from build123d import *

# Parameters (mm, degrees)
SKETCH1_W           = 80
SKETCH1_H           = 15
BOSS_EXTRUDE1_DEPTH = 5
FILLET1_R           = 6
SKETCH3_W           = 20
SKETCH3_H           = 15
CUT_EXTRUDE2_DEPTH  = 2.5
CUT_EXTRUDE3_DEPTH  = 2
SKETCH5_R           = 1.25
CUT_EXTRUDE4_DEPTH  = 41.807474805
SKETCH6_R           = 2.5
CUT_EXTRUDE5_DEPTH  = 1.5
SKETCH7_R           = 3.677678073
CUT_EXTRUDE6_DEPTH  = 1


with BuildPart() as part:
    # Sketch1 → Boss-Extrude1 (new body)
    with BuildSketch(Plane(origin=(0, 0, 0), x_dir=(1, 0, 0), z_dir=(0, 1, 0))):
        Rectangle(SKETCH1_W, SKETCH1_H)
    extrude(amount=BOSS_EXTRUDE1_DEPTH)

    # Fillet1
    fillet1_edges = [part.edges().sort_by_distance(p)[0] for p in [
        (-40, 2.5, -7.5),
        (40, 2.5, -7.5),
        (40, 2.5, 7.5),
        (-40, 2.5, 7.5),
    ]]
    fillet(fillet1_edges, radius=FILLET1_R)

    # Sketch3 → Cut-Extrude2 (cut)
    with BuildSketch(Plane(origin=(0, 5, 0), x_dir=(1, 0, 0), z_dir=(0, 1, 0))):
        with Locations((20.062463618, 0)):
            Rectangle(SKETCH3_W, SKETCH3_H)
    extrude(amount=-CUT_EXTRUDE2_DEPTH, mode=Mode.SUBTRACT)

    # Sketch4 → Cut-Extrude3 (cut)
    with BuildSketch(Plane(origin=(0, 5, 0), x_dir=(1, 0, 0), z_dir=(0, 1, 0))):
        with BuildLine():
            Line((-20.5, 3.7), (-6, 2.1))
            ThreePointArc((-6, 2.1), (-3.9, 0), (-6, -2.1))
            Line((-6, -2.1), (-20.5, -3.7))
            Line((-20.5, -3.7), (-35, -2.1))
            ThreePointArc((-35, -2.1), (-37.1, 0), (-35, 2.1))
            Line((-35, 2.1), (-20.5, 3.7))
        make_face()
    extrude(amount=-CUT_EXTRUDE3_DEPTH, mode=Mode.SUBTRACT)

    # Sketch5 → Cut-Extrude4 (cut, through all)
    with BuildSketch(Plane(origin=(0, 3, 0), x_dir=(1, 0, 0), z_dir=(0, 1, 0))):
        with Locations(Location((-20.5, 0, 0), (0, 0, 270))):
            Circle(SKETCH5_R)
    extrude(amount=-CUT_EXTRUDE4_DEPTH, mode=Mode.SUBTRACT)

    # Sketch6 → Cut-Extrude5 (cut)
    with BuildSketch(Plane(origin=(0, 0, 0), x_dir=(-1, 0, 0), z_dir=(0, -1, 0))):
        with Locations(Location((20.5, 0, 0), (0, 0, 90))):
            Circle(SKETCH6_R)
    extrude(amount=-CUT_EXTRUDE5_DEPTH, mode=Mode.SUBTRACT)

    # Sketch7 → Cut-Extrude6 (cut)
    with BuildSketch(Plane(origin=(0, 3, 0), x_dir=(1, 0, 0), z_dir=(0, 1, 0))):
        with Locations(Location((-20.5, 0, 0), (0, 0, 270))):
            Circle(SKETCH7_R)
    extrude(amount=-CUT_EXTRUDE6_DEPTH, mode=Mode.SUBTRACT)


solid = part.part
Can you work these out from the model? Positions are in its coordinate system, mm. A direction names the side the tool comes from. Coordinates: 2 decimals unless noted, no trailing zeros. Write each loop counter-clockwise with the first axis right and the second up, starting at its lowest first coordinate (ties: lowest second). Pieces come first, ordered by that corner, then holes.
Q1. If we mould it in two halves opening along X, with no side actions, what happens to faces 1 (the face through (-38.289, 2.535, -5.696)), 2 (the face through (-27.85, 4.01, -2.89)), 3 (the face through (40, 2, 0))? For each: +X half, -X half, draft (parallel to the pull), parting line (faces both ways), or undercut.
Results found:
face 1: -X half
face 2: undercut
face 3: +X half
Q2. Imagine slicing it at B-B, the plane z = 0. List the corners of the cut face in (x, y) for me.
Results found:
outline: (-40, 0) - (-23, 0) - (-23, 1.5) - (-21.75, 1.5) - (-21.75, 2) - (-24.18, 2) - (-24.18, 3) - (-37.1, 3) - (-37.1, 5) - (-40, 5) - close; (-19.25, 1.5) - (-18, 1.5) - (-18, 0) - (40, 0) - (40, 5) - (30.06, 5) - (30.06, 2.5) - (10.06, 2.5) - (10.06, 5) - (-3.9, 5) - (-3.9, 3) - (-16.82, 3) - (-16.82, 2) - (-19.25, 2) - close
Q3. Which directions (+Z, -Z, +X, -X, +Y, -Y) give clear straight access to the entire face, cutting with the end or side of a thin tool? Please do faces 4 (the face through (35, 5, 0)), 5 (the face through (30.062, 4, 0)), 6 (the face through (-22, 2, 0)), 7 (the face through (-18, 1, 0)).
Results found:
face 4: +Z, -Z, +X, -X, +Y
face 5: +Z, -Z, +Y
face 6: +Y
face 7: -Y
Q4. For P1, Ø1.5, axis at y = 4.5, z = 3.5, coming from the -X side; P2, Ø2, axis at y = 4, z = 4.5, coming from the +X side; P3, Ø4.5, axis at x = -20.5, z = 0, coming from the +Y side, each with a flat end and sliding along its axis, tell me the tip position at first contact or that it passes through.
Results found:
P1: stops at x = -39.87
P2: stops at x = 39.66
P3: stops at y = 2
Q5. Imagine slicing it at A-A, the plane y = 3.9. List the corners of the cut face in (x, z) for me.
Results found:
outline: (-40, -1.5) arc R6 ccw to (-34, -7.5) - (10.06, -7.5) - (10.06, 7.5) - (-34, 7.5) arc R6 ccw to (-40, 1.5) - close; (30.06, -7.5) - (34, -7.5) arc R6 ccw to (40, -1.5) - (40, 1.5) arc R6 ccw to (34, 7.5) - (30.06, 7.5) - close; hole (-35, -2.1) - (-20.5, -3.7) - (-6, -2.1) arc R2.1 ccw to (-6, 2.1) - (-20.5, 3.7) - (-35, 2.1) arc R2.1 ccw to start
Q6. Imagine slicing it at D-D, the plane x = -13. List the corners of the cut face in (y, z) for me.
Results found:
outline: (0, -7.5) - (5, -7.5) - (5, -2.87) - (3, -2.87) - (3, 2.87) - (5, 2.87) - (5, 7.5) - (0, 7.5) - close
Q7. Imagine slicing it at C-C, the plane z = 5.75. List the corners of the cut face in (x, y) for me.
Results found:
outline: (-38.24, 0) - (38.24, 0) - (38.24, 5) - (30.06, 5) - (30.06, 2.5) - (10.06, 2.5) - (10.06, 5) - (-38.24, 5) - close
Q8. Please list where these lines run through material, in increasing order: L1, parallel to X at y = 1.8, z = 0; L2, parallel to X at y = 4.8, z = -0.5; L3, parallel to X at y = 4.35, z = 1.25.
Results found:
L1: x = -40 to -21.75, -19.25 to 40
L2: x = -40 to -37.04, -3.96 to 10.06, 30.06 to 40
L3: x = -40 to -36.69, -4.31 to 10.06, 30.06 to 40
